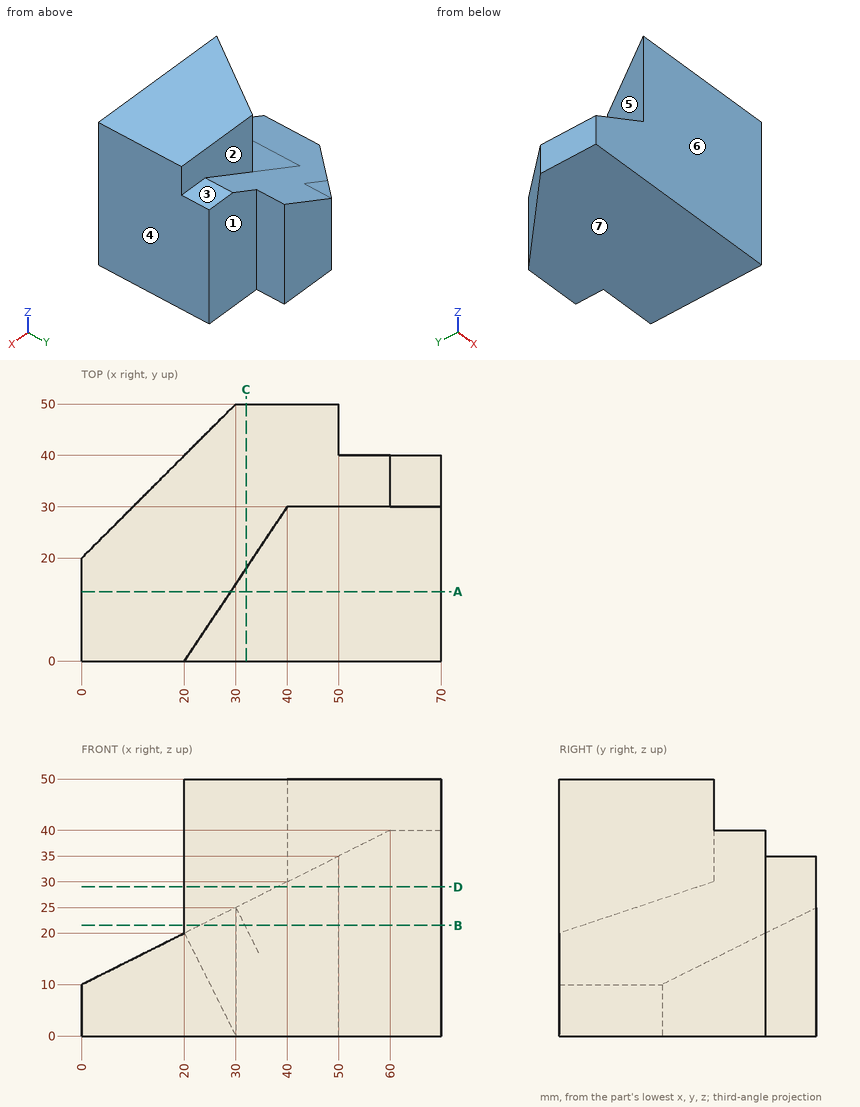
Geometry check sheet. Reference: drawing and pictorial views, mm from the part's lowest x, y, z. A direction names the side the tool comes from. Give positions to 0.01 mm unless a question says otherwise; leave off trailing zeros. Loops run counter-clockwise (first coordinate to the right, second up) from the corner with the lowest first, then second, coordinate; pieces in that order, holes last.
1. Go/stop test with flat-tipped pins: pin 1 Ø3 at (y, z) = (45, 13) entering from +X; pin 2 Ø12 at (x, z) = (18.5, 17) entering from +Y; pin 3 Ø3 at (y, z) = (39, 9) entering from -X. Record where each tip stops, or that it passes through.
2. Thickness scan on line 1 (Y direction, x = 51, z = 30); line 2 (Y direction, x = 50, z = 45). Record the ranges inside material, lowest first.
3. Mould release check, pull along Y, two halves, no side actions. Record for the marked faces 5, 6 and 7: released by +Y, released by -Y, zero draft, split by the parting line, or undercut.
4. Set-up check for the marked faces 1, 2, 3 and 4: record each of +Z, -Z, +X, -X, +Y, -Y from which the full face is reachable in a straight line by a thin tool's end or side.
5. Section check D-D, the plane z = 29. Enter the section's corners in (x, y), then the cut area to 3 significant figures.
6. Section check C-C, the plane x = 32. Enter the section's corners in (y, z).
7. Section check A-A, the plane y = 13.5. Enter the section's corners in (x, z), then the cut area to 3 significant figures.
8. Section check B-B, the plane z = 21.5. Enter the section's corners in (x, y).
Geometry says:
1. pin 1: stops at x = 50
1. pin 2: stops at y = 44.5
1. pin 3: stops at x = 17.5
2. line 1: y = 0 to 40
2. line 2: y = 0 to 30
3. face 5: released by +Y
3. face 6: released by -Y
3. face 7: zero draft
4. face 1: +Z, -Z, +X, +Y
4. face 2: +Z, -X, +Y
4. face 3: +Z, +X, -X, +Y
4. face 4: +Z, -Z, +X, +Y, -Y
5. outline: (20, 0) - (70, 0) - (70, 40) - (50, 40) - (50, 50) - (38, 50) - (38, 27) - close
5. area: 1,640 mm2
6. outline: (0, 0) - (50, 0) - (50, 26) - (18, 26) - (18, 50) - (0, 50) - close
7. outline: (0, 0) - (70, 0) - (70, 50) - (29, 50) - (29, 24.5) - (0, 10) - close
7. area: 2,550 mm2
8. outline: (20, 0) - (70, 0) - (70, 40) - (50, 40) - (50, 50) - (30, 50) - (23, 43) - (23, 4.5) - close
